CAD build for the part. Positions are in the model's coordinates, mm. A direction names the side the tool comes from. Round coordinates to 2 decimals unless told otherwise and drop trailing zeros. Write each loop counter-clockwise with the first axis right and the second up, starting at its lowest first coordinate (ties: lowest second). Pieces come first, ordered by that corner, then holes. Notation, with made-up numbers: (-15, 50) - (21, 50) arc R25 ccw to (21, 69) - close; hole circle Ø5 at (-40, -2.5). An arc over 180 degrees is marked (long way). Answer in a Markdown table with one row per item.
```python
from build123d import *

# Parameters (mm, degrees)
SKETCH1_W           = 55.626
SKETCH1_H           = 139.7
BOSS_EXTRUDE1_DEPTH = 35.56
CUT_EXTRUDE1_DEPTH  = 27.94
CUT_EXTRUDE6_DEPTH  = 30.48
SKETCH4_R           = 3.175
CUT_EXTRUDE7_DEPTH  = 155.514903734
SKETCH5_W           = 12.7
SKETCH5_H           = 12.7
CUT_EXTRUDE8_DEPTH  = 140.273747309
BOSS_EXTRUDE2_DEPTH = 83.82
SKETCH7_W           = 20.32
SKETCH7_H           = 30.48
SKETCH7_R           = 6.35
BOSS_EXTRUDE3_DEPTH = 3.175
SKETCH8_W           = 6.35
SKETCH8_H           = 83.82
CUT_EXTRUDE9_DEPTH  = 17.78
FILLET1_R           = 7.62
FILLET2_R           = 2.54
FILLET3_R           = 1.27


with BuildPart() as part:
    # Sketch1 → Boss-Extrude1 (new body)
    with BuildSketch(Plane.XY):
        with Locations((27.813, -69.85)):
            Rectangle(SKETCH1_W, SKETCH1_H)
    extrude(amount=BOSS_EXTRUDE1_DEPTH)

    # Sketch2 → Cut-Extrude1 (cut)
    with BuildSketch(Plane(origin=(0, 0, 5.08), x_dir=(-1, 0, 0), z_dir=(0, 0, -1))):
        Polygon((-1.778, -33.02), (-53.848, -33.02), (-53.848, -122.6312), (-41.148, -122.6312), (-41.148, -139.7), (-14.478, -139.7), (-14.478, -122.6312), (-1.778, -122.6312), align=None)
    extrude(amount=-CUT_EXTRUDE1_DEPTH, mode=Mode.SUBTRACT)

    # Sketch3 → Cut-Extrude6 (cut)
    with BuildSketch(Plane.XY.offset(35.56)):
        Polygon((24.003, -139.7), (31.623, -139.7), (31.623, -76.2), (53.848, -76.2), (53.848, 0), (1.778, 0), (1.778, -76.2), (24.003, -76.2), align=None)
    extrude(amount=-CUT_EXTRUDE6_DEPTH, mode=Mode.SUBTRACT)

    # Sketch4 → Cut-Extrude7 (cut, through all)
    with BuildSketch(Plane(origin=(0, 0, 0), x_dir=(-1, 0, 0), z_dir=(0, 0, -1))):
        with Locations((-27.813, -5.588)):
            Circle(SKETCH4_R)
    extrude(amount=-CUT_EXTRUDE7_DEPTH, mode=Mode.SUBTRACT)

    # Sketch5 → Cut-Extrude8 (cut, through all)
    with BuildSketch(Plane(origin=(0, -122.6312, 0), x_dir=(1, 0, 0), z_dir=(0, 1, 0))):
        with Locations((8.128, -11.43)):
            Rectangle(SKETCH5_W, SKETCH5_H)
        with Locations((47.498, -26.67)):
            Rectangle(SKETCH5_W, SKETCH5_H)
    extrude(amount=-CUT_EXTRUDE8_DEPTH, mode=Mode.SUBTRACT)

    # Sketch6 → Boss-Extrude2 (add)
    with BuildSketch(Plane.XZ.offset(139.7)):
        Polygon((55.626, 0), (78.486, 0), (78.486, 35.56), (55.626, 35.56), (55.626, 33.02), (75.946, 33.02), (75.946, 2.54), (55.626, 2.54), align=None)
    extrude(amount=-BOSS_EXTRUDE2_DEPTH)

    # Sketch7 → Boss-Extrude3 (add)
    with BuildSketch(Plane.XZ.offset(139.7)):
        with Locations((65.786, 17.78)):
            Rectangle(SKETCH7_W, SKETCH7_H)
        with Locations(Location((64.262, 17.78, 0), (0, 0, 270))):
            Circle(SKETCH7_R, mode=Mode.SUBTRACT)
    extrude(amount=-BOSS_EXTRUDE3_DEPTH)

    # Sketch8 → Cut-Extrude9 (cut)
    with BuildSketch(Plane.XY.offset(35.56)):
        with Locations((64.262, -97.79)):
            Rectangle(SKETCH8_W, SKETCH8_H)
    extrude(amount=-CUT_EXTRUDE9_DEPTH, mode=Mode.SUBTRACT)

    # Fillet1
    fillet1_edges = [part.edges().sort_by_distance(p)[0] for p in [
        (67.437, -138.1125, 23.279261314),
        (61.087, -138.1125, 23.279261314),
        (54.737, 0, 35.56),
        (14.478, -131.1656, 33.02),
        (41.148, -131.1656, 5.08),
        (0.889, 0, 35.56),
    ]]
    fillet(fillet1_edges, radius=FILLET1_R)

    # Fillet2
    fillet2_edges = [part.edges().sort_by_distance(p)[0] for p in [
        (53.848, -131.1656, 20.32),
        (41.148, -131.1656, 20.32),
        (55.626, -96.2025, 2.54),
        (75.946, -96.2025, 2.54),
        (75.946, -96.2025, 33.02),
        (55.626, -96.2025, 33.02),
        (55.626, -136.525, 17.78),
        (71.6915, -136.525, 33.02),
        (75.946, -136.525, 17.78),
        (65.786, -136.525, 2.54),
        (58.3565, -136.525, 33.02),
        (61.087, -55.88, 34.29),
        (67.437, -55.88, 34.29),
        (1.778, -99.4156, 33.02),
        (11.938, -122.6312, 33.02),
        (1.778, -122.6312, 25.4),
        (43.688, -122.6312, 5.08),
        (1.778, -69.85, 5.08),
        (53.848, -61.3156, 5.08),
        (53.848, -107.95, 33.02),
        (12.8905, -76.2, 33.02),
        (1.778, -76.2, 34.29),
        (42.7355, -76.2, 33.02),
        (24.003, -76.2, 34.29),
        (53.848, -76.2, 34.29),
        (31.623, -76.2, 34.29),
        (53.848, -122.6312, 12.7),
        (1.778, -131.1656, 17.78),
        (14.478, -131.1656, 17.78),
    ]]
    fillet(fillet2_edges, radius=FILLET2_R - 0.0001)  # a hair under: the kernel refuses the full size

    # Fillet3
    fillet3_edges = [part.edges().sort_by_distance(p)[0] for p in [
        (55.626, -31.75, 35.56),
        (78.486, -97.79, 35.56),
        (72.9615, -139.7, 35.56),
        (55.626, 0, 13.97),
        (0, 0, 13.97),
        (55.626, -2.231846327, 33.328153673),
        (0, -73.66, 35.56),
        (0, -2.231846327, 33.328153673),
        (46.355, -139.7, 35.56),
        (0, -139.7, 17.78),
        (12.0015, -139.7, 35.56),
    ]]
    fillet(fillet3_edges, radius=FILLET3_R)


solid = part.part
```
Q1. Flat gauge pins, fed straight in: pin 1 (23.5 mm diameter, centred on x = 18, y = -61.5, fed in from +Z); pin 2 (4 mm diameter, centred on y = -42.5, z = 19.5, fed in from +X); pin 3 (7.5 mm diameter, centred on x = 64.262, z = 17.78, fed in from -Y); pin 4 (3.5 mm diameter, centred on x = 47, z = 16.5, fed in from +Y). Where does each tip first touch, or does it go through?
Computed:
| item | result |
|---|---|
| pin 1 | stops at z = 5.08 |
| pin 2 | stops at x = 55.63 |
| pin 3 | passes through |
| pin 4 | stops at y = -122.63 |
Q2. Saw through at A-A on y = -62.5. List the corners of the cut face in (x, z), then the cut area to 3 significant figures.
Computed:
| item | result |
|---|---|
| outline | (0, 0) - (78.49, 0) - (78.49, 34.29) arc R1.27 ccw to (77.22, 35.56) - (67.44, 35.56) - (67.44, 33.02) - (73.41, 33.02) arc R2.54 cw to (75.95, 30.48) - (75.95, 5.08) arc R2.54 cw to (73.41, 2.54) - (58.17, 2.54) arc R2.54 cw to (55.63, 5.08) - (55.63, 30.48) arc R2.54 cw to (58.17, 33.02) - (61.09, 33.02) - (61.09, 35.56) - (53.85, 35.56) - (53.85, 7.62) arc R2.54 cw to (51.31, 5.08) - (4.32, 5.08) arc R2.54 cw to (1.78, 7.62) - (1.78, 35.56) - (1.27, 35.56) arc R1.27 ccw to (0, 34.29) - close |
| area | 576 mm2 |
Q3. Pull direction X, two halves, no side cores. Call faces 1 (the flat face through (69, -136.525, 12)), 2 (the flat face through (70, -95, 33.02)), 3 (the flat face through (72, -98, 35.56)): released by +X, released by -X, zero draft, split by the parting line, or undercut.
Computed:
| item | result |
|---|---|
| face 1 | undercut |
| face 2 | undercut |
| face 3 | zero draft |
Q4. 3-axis set-ups, long thin cutter, end or side, ignore diameter. For faces 4 (the flat face through (9, -122.631, 24)), 5 (the cylindrical face through (68.201, -56.604, 34.272)), 6 (the cylindrical face through (16.65, -129.76, 30.73)), 7 (the flat face through (61.087, -102, 34)): which of +Z, -Z, +X, -X, +Y, -Y reach the whole face in a straight line?
Computed:
| item | result |
|---|---|
| face 4 | +Y |
| face 5 | +Z, +Y |
| face 6 | +Y, -Y |
| face 7 | +Z, +Y, -Y |
Q5. Drill centre lines: line 1 (X direction, y = -60, z = 14); line 2 (X direction, y = -93, z = 33.5); line 3 (Z direction, x = 18, y = -83). Where is each one in solid material? Low to high.
Computed:
| item | result |
|---|---|
| line 1 | x = 0 to 1.78, 53.85 to 55.63, 75.95 to 78.49 |
| line 2 | x = 0 to 24, 31.62 to 61.09, 67.44 to 78.49 |
| line 3 | z = 0 to 5.08, 33.02 to 35.56 |
